```python
from build123d import *

# Parameters (mm, degrees)
F0_R     = 4
F1_DEPTH = 16
F3_DEPTH = 5.3
F4_R     = 5
F5_DEPTH = 1


with BuildPart() as f1:
    # F0 (on Top) → F1 (new body)
    with BuildSketch(Plane.XY):
        Circle(F0_R)
    extrude(amount=F1_DEPTH)

    # F2 (on face) → F3 (join)
    with BuildSketch(Plane.XY.offset(16)):
        Polygon((3.781678, -6.483228), (7.505479, 0.033416), (3.723801, 6.516643), (-3.781678, 6.483228), (-7.505479, -0.033416), (-3.723801, -6.516643), align=None)
    extrude(amount=F3_DEPTH)

    # F4 (on face) → F5 (cut)
    with BuildSketch(Plane(origin=(0, 0, 16), x_dir=(1, 0, 0), z_dir=(0, 0, -1))):
        Polygon((3.723801, -6.516643), (7.505479, -0.033416), (3.781678, 6.483228), (-3.723801, 6.516643), (-7.505479, 0.033416), (-3.781678, -6.483228), align=None)
        Circle(F4_R, mode=Mode.SUBTRACT)
    extrude(amount=-F5_DEPTH, mode=Mode.SUBTRACT)


solid = f1.part
```
For this review, take the finished solid that the model builds, in its own axes (mm). A direction names the side the tool comes from. Round coordinates to 2 decimals unless told otherwise and drop trailing zeros. Loops run counter-clockwise (first coordinate to the right, second up) from the corner with the lowest first, then second, coordinate; pieces in that order, holes last.
(1) We need section A-A (z = 18.5). Give the boundary of the cut face in (x, y).
Returned:
outline: (-7.51, -0.03) - (-3.72, -6.52) - (3.78, -6.48) - (7.51, 0.03) - (3.72, 6.52) - (-3.78, 6.48) - close
(2) We need section C-C (y = -2.75). Give the boundary of the cut face in (x, z), plus the area to 3 significant figures.
Returned:
outline: (-5.92, 17) - (-4.18, 17) - (-4.18, 16) - (-2.9, 16) - (-2.9, 0) - (2.9, 0) - (2.9, 16) - (4.18, 16) - (4.18, 17) - (5.91, 17) - (5.91, 21.3) - (-5.92, 21.3) - close
area: 152 mm2
(3) Tool access review of faces 1 (the flat face through (4.4, 2.9, 17)), 2 (the flat face through (-5.6, 3.3, 19.1)): name each direction out of +Z, -Z, +X, -X, +Y, -Y from which nothing blocks a thin tool from reaching the whole face with its end or side.
Returned:
face 1: -Z
face 2: +Z, -Z, -X, +Y
(4) We need section B-B (x = 0). Give the boundary of the cut face in (y, z).
Returned:
outline: (-6.5, 17) - (-5, 17) - (-5, 16) - (-4, 16) - (-4, 0) - (4, 0) - (4, 16) - (5, 16) - (5, 17) - (6.5, 17) - (6.5, 21.3) - (-6.5, 21.3) - close
(5) We need section D-D (z = 2.5). Give the boundary of the cut face in (x, y), plus the area to 3 significant figures.
Returned:
outline: circle Ø8 at (0, 0)
area: 50.3 mm2
(6) Clearance check with flat-ended pins moving along their axes: P1, Ø6, axis at x = -4, z = 5, coming from the -Y side; P2, Ø1, axis at x = -4, z = 15, coming from the -Y side; P3, Ø5, axis at y = -2, z = 6, coming from the -X side. State where each tip first meets the part, or that it passes through.
Returned:
P1: stops at y = -3.87
P2: stops at y = -1.94
P3: stops at x = -4
(7) Wall thickness on line 1 along Z through (x, y) = (-5, 3.5); line 2 along Y through (x, z) = (3.25, 20.5); line 3 along X through (y, z) = (3, 10.5): over which ranges is each line inside the solid? List them lowest first.
Returned:
line 1: z = 17 to 21.3
line 2: y = -6.49 to 6.51
line 3: x = -2.65 to 2.65
